Could you check a few things on this model? Use its own coordinates, in mm. A direction names the side the tool comes from. Give positions to 0.01 mm unless a question says otherwise; leave off trailing zeros. Write each loop counter-clockwise with the first axis right and the second up, starting at its lowest first coordinate (ties: lowest second). Pieces come first, ordered by that corner, then holes. Notation, with made-up numbers: (-2, -37.75) -> (17, -37.75) arc R14 cw to (17, -30.75) -> close; hole circle Ø7 at (0.5, 0). An arc over 180 degrees is marked (long way). Write item = value, one per line. Start each with the question number.
Autodesk Fusion 360 part; units mm, degrees
sketch "Sketch1" plane through (0, 0, 0) normal (0, 1, 0) x (1, 0, 0)
  line L0 (7.8, -3.815) -> (-7.8, -3.815)
  line L1 (-7.8, -3.815) -> (-7.8, 3.815)
  line L2 (-7.8, 3.815) -> (7.8, 3.815)
  line L3 (7.8, 3.815) -> (7.8, -3.815)
  line L4 (7.8, -3.815) -> (-7.8, 3.815) construction
  line L5 (-7.8, -3.815) -> (7.8, 3.815) construction
  line L6 (8.225, -4.25) -> (-8.225, -4.25)
  line L7 (-8.225, -4.25) -> (-8.225, 4.25)
  line L8 (-8.225, 4.25) -> (8.225, 4.25)
  line L9 (8.225, 4.25) -> (8.225, -4.25)
  line L10 (8.225, -4.25) -> (-8.225, 4.25) construction
  line L11 (-8.225, -4.25) -> (8.225, 4.25)
  line L12 (12.5, -7.5) -> (-12.5, -7.5)
  line L13 (-12.5, -7.5) -> (-12.5, 7.5)
  line L14 (-12.5, 7.5) -> (12.5, 7.5)
  line L15 (12.5, 7.5) -> (12.5, -7.5)
  line L16 (12.5, -7.5) -> (-12.5, 7.5) construction
  line L17 (-12.5, -7.5) -> (12.5, 7.5) construction
  dimension "d1" = 15.6
  dimension "d2" = 7.63
  dimension "d3" = 16.45
  dimension "d4" = 8.5
  dimension "d5" = 25
  dimension "d6" = 15
extrude "Extrude1" add sketch "Sketch1" against normal blind 12.25 makes body 1
extrude "Extrude2" add sketch "Sketch1" along normal blind 4 contours L0 L2 L3 L6 L9 L11 | L0 L1 L2 L7 L8 L11 | L12 L13 L14 L15 bodies 1
copy_body "Body->Comp1" bodies 1 removing the originals makes body 2 in component "PairHolder"
component "PairHolder" placed x (1, 0, 0) y (0, 1, 0) z (0, 0, 1) at (0, 0, 0)
(1) We'd pull the mould along X, two halves only. Please class faces 4 (the flat face through (8.225, -6, 0)), 5 (the flat face through (0, -12.25, -5)), 6 (the flat face through (12.5, -4, 0)): released by +X, released by -X, zero draft, split by the parting line, or undercut.
(2) Imagine slicing it at D-D (y = 1.25). Please give me the cut outline in (x, z) (3 decimals).
(3) If I drill on line 1 along X through (y, z) = (-6.75, -3.25) (3 decimals); line 2 along Z through (x, y) = (6.75, -8); line 3 along X through (y, z) = (0.25, 0), over which ranges is the centre line in solid material (lowest first)? Write a range as from..to.
(4) Imagine slicing it at C-C (z = -3.5). Please give me the cut outline in (x, y) (3 decimals), then the cut area to 3 significant figures.
(5) Imagine slicing it at B-B (x = -1.5). Please give me the cut outline in (y, z) (3 decimals).
(6) On a 3-axis mill with a long thin cutter (end or side, diameter ignored), from which of +Z, -Z, +X, -X, +Y, -Y can I reach the whole of each face in a straight line? I mean faces 1 (the flat face through (0, 2, -3.815)), 2 (the flat face through (0, -4, -7.5)), 3 (the flat face through (0, -6, -4.25)). Say none if no direction works.
(7) Imagine slicing it at A-A (y = -0.5). Please give me the cut outline in (x, z) (3 decimals).
Answers below:
q1.face_4 = undercut
q1.face_5 = zero draft
q1.face_6 = released by +X
q2.outline = (-12.5, -7.5) -> (12.5, -7.5) -> (12.5, 7.5) -> (-12.5, 7.5) -> close; hole (-7.8, -3.815) -> (7.8, -3.815) -> (7.8, 3.815) -> (-7.8, 3.815) -> close
q3.line_1 = -12.5..-8.225, 8.225..12.5
q3.line_2 = -7.5..-4.25, 4.25..7.5
q3.line_3 = -12.5..-7.8, 7.8..12.5
q4.outline = (-12.5, -12.25) -> (-8.225, -12.25) -> (-8.225, 0) -> (-7.8, 0) -> (-7.8, 4) -> (-12.5, 4) -> close; (7.8, 0) -> (8.225, 0) -> (8.225, -12.25) -> (12.5, -12.25) -> (12.5, 4) -> (7.8, 4) -> close
q4.area = 142 mm^2
q5.outline = (-12.25, -7.5) -> (4, -7.5) -> (4, -3.815) -> (0, -3.815) -> (0, -4.25) -> (-12.25, -4.25) -> close; (-12.25, 4.25) -> (0, 4.25) -> (0, 3.815) -> (4, 3.815) -> (4, 7.5) -> (-12.25, 7.5) -> close
q6.face_1 = +Y, -Y
q6.face_2 = -Z, +X, -X, +Y, -Y
q6.face_3 = -Y
q7.outline = (-12.5, -7.5) -> (12.5, -7.5) -> (12.5, 7.5) -> (-12.5, 7.5) -> close; hole (-8.225, -4.25) -> (8.225, -4.25) -> (8.225, 4.25) -> (-8.225, 4.25) -> close
